The listing builds one solid part. Answer for the finished solid, in the listing's coordinates (mm). Round coordinates to 2 decimals unless told otherwise and drop trailing zeros. Write each loop counter-clockwise with the first axis right and the second up, starting at its lowest first coordinate (ties: lowest second). Pieces come first, ordered by that corner, then holes. Notation, with made-up numbers: (71, 3.5) - (106, 3.5) arc R22 ccw to (106, 32.5) - close; hole circle Ø10 at (76, 65). An arc over 180 degrees is marked (long way). Return JSON: item names as keys, results as strings. Group by question number.
(1) Each of these flat-tipped pins is pushed along its axis until it touches: pin 1 (12 mm diameter, centred on x = 37.5, y = -10, fed in from -Z); pin 2 (3 mm diameter, centred on x = -447.5, z = 5.5, fed in from -Y); pin 3 (1 mm diameter, centred on y = -12, z = 11, fed in from +X); pin 4 (5 mm diameter, centred on x = -548, z = 16, fed in from +Y). Where does it stop, or does it pass through?
(2) Find the intervals of material crossed by line 1 along X through (y, z) = (0, -18.55) (3 decimals); line 2 along Y through (x, z) = (-280, 0); line 3 along Z through (x, y) = (-164.5, 2.5), in increasing order. Write a range as [from, to].
(3) Section A-A, the plane z = 0 is taken. Write down the section's boundary in (x, y), then the cut area to 3 significant figures.
(4) Section B-B, the plane x = 742 is taken. Write down the section's boundary in (y, z), then the cut area to 3 significant figures.
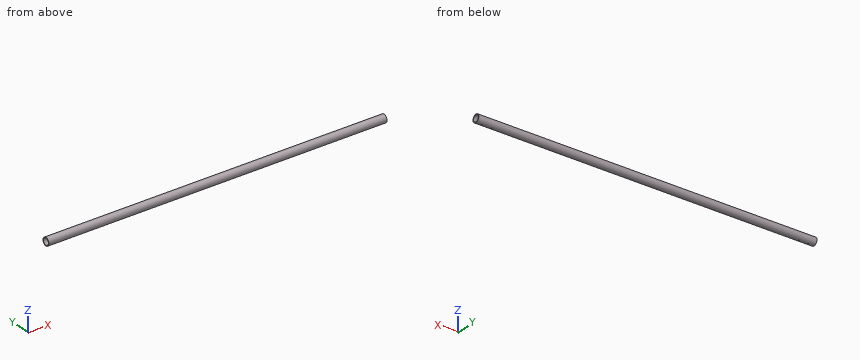
```python
from build123d import *

# Parameters (mm, degrees)
SKETCH1_R                = 21.082
SKETCH1_R_2              = 17.526
BOSS_EXTRUDE1_DEPTH      = 914.4
BOSS_EXTRUDE1_DEPTH_BACK = 914.4
SKETCH2_R                = 3.175
CUT_EXTRUDE1_DEPTH       = 22.082


with BuildPart() as part:
    # Sketch1 → Boss-Extrude1 (new body, two sides)
    with BuildSketch(Plane(origin=(0, 0, 0), x_dir=(0, 0, -1), z_dir=(1, 0, 0))) as boss_extrude1_sk:
        Circle(SKETCH1_R)
        Circle(SKETCH1_R_2, mode=Mode.SUBTRACT)
    extrude(amount=BOSS_EXTRUDE1_DEPTH)
    extrude(boss_extrude1_sk.sketch, amount=-BOSS_EXTRUDE1_DEPTH_BACK)

    # Sketch2 → Cut-Extrude1 (cut, through all)
    with BuildSketch(Plane.XY):
        with Locations((-831.85, 0)):
            Circle(SKETCH2_R)
        with Locations((-882.65, 0)):
            Circle(SKETCH2_R)
    cut_extrude1 = extrude(amount=-CUT_EXTRUDE1_DEPTH, mode=Mode.SUBTRACT)

    # Mirror1: Cut-Extrude1 across plane
    add(cut_extrude1.mirror(Plane(origin=(0, 0, 0), x_dir=(0, 0, 1), z_dir=(1, 0, 0))), mode=Mode.SUBTRACT)


solid = part.part
```
Working result:
{
 "1": {"pin 1": "stops at z = -20.7", "pin 2": "stops at y = -20.7", "pin 3": "passes through", "pin 4": "stops at y = 16.19"},
 "2": {"line 1": "x = [-914.4, -885.825], [-879.475, -835.025], [-828.675, 828.675], [835.025, 879.475], [885.825, 914.4]", "line 2": "y = [-21.08, -17.53], [17.53, 21.08]", "line 3": "z = [-20.93, -17.35], [17.35, 20.93]"},
 "3": {"outline": "(-914.4, -21.08) - (914.4, -21.08) - (914.4, -17.53) - (-914.4, -17.53) - close; (-914.4, 17.53) - (914.4, 17.53) - (914.4, 21.08) - (-914.4, 21.08) - close", "area": "13,000 mm^2"},
 "4": {"outline": "circle Ø42.16 at (0, 0); hole circle Ø35.05 at (0, 0)", "area": "431 mm^2"}
}
